Work out the finished part from the listing and answer in its coordinate system (mm). Face numbers are marked on the shaded views. A direction names the side the tool comes from. Coordinates: 2 decimals unless noted, no trailing zeros. Loops run counter-clockwise (first coordinate to the right, second up) from the corner with the lowest first, then second, coordinate; pieces in that order, holes last. Notation, with made-up numbers: (58, -39) -> (78, -39) arc R26 cw to (78, -13) -> close; hole circle Ø11 at (74, 45). An arc over 180 degrees is marked (long way). Answer as CSV lines item,"result".
Autodesk Fusion 360 part; units mm, degrees
sketch "Sketch1" plane through (0, 0, 0) normal (0, 0, 1) x (1, 0, 0)
  line L0 (49.35, -38.85) -> (-49.35, -38.85)
  line L1 (-49.35, -38.85) -> (-49.35, 38.85)
  line L2 (-49.35, 38.85) -> (49.35, 38.85)
  line L3 (49.35, 38.85) -> (49.35, -38.85)
  line L4 (49.35, -38.85) -> (-49.35, 38.85) construction
  line L5 (-49.35, -38.85) -> (49.35, 38.85) construction
  dimension "d1" = 98.7
  dimension "d2" = 77.7
extrude "Extrude1" add sketch "Sketch1" along normal blind 4
sketch "Sketch2" plane through (0, 0, 4) normal (0, 0, 1) x (-1, 0, 0)
  line L0 (-49.35, -38.85) -> (49.35, -38.85)
  line L1 (49.35, -38.85) -> (49.35, 38.85)
  line L2 (49.35, 38.85) -> (-49.35, 38.85)
  line L3 (-49.35, 38.85) -> (-49.35, -38.85)
  line L4 (35.35, -38.85) -> (-34.25, -38.85)
  line L5 (-34.25, -38.85) -> (-34.25, 9.95)
  line L6 (-34.25, 9.95) -> (35.35, 9.95)
  line L7 (35.35, 9.95) -> (35.35, -38.85)
  dimension "d5" = 69.6
  dimension "d6" = 48.8
  dimension "d7" = 14
extrude "Extrude2" add sketch "Sketch2" along normal blind 10 contours L0 L4 L5 L6 L7
sketch "Sketch3" plane through (0, 0, 14) normal (0, 0, 1) x (-1, 0, 0)
  line L0 (35.35, 9.95) -> (-34.25, 9.95)
  line L1 (-34.25, 9.95) -> (-34.25, -38.85)
  line L2 (-34.25, -38.85) -> (35.35, -38.85)
  line L3 (35.35, -38.85) -> (35.35, 9.95)
  line L4 (30.35, -38.85) -> (-28.35, -38.85)
  line L5 (-28.35, -38.85) -> (-28.35, 0.45)
  line L6 (-28.35, 0.45) -> (30.35, 0.45)
  line L7 (30.35, 0.45) -> (30.35, -38.85)
  dimension "d10" = 39.3
  dimension "d11" = 58.7
  dimension "d12" = 5
extrude "Extrude3" add sketch "Sketch3" along normal blind 20 contours L2 L4 L5 L6 L7
sketch "Sketch4" plane through (0, 0, 4) normal (0, 0, 1) x (-1, 0, 0)
  line L0 (-34.25, -38.85) -> (-34.25, 9.95)
  line L1 (-34.25, 9.95) -> (35.35, 9.95)
  line L2 (35.35, 9.95) -> (35.35, -38.85)
  line L3 (35.35, -38.85) -> (49.35, -38.85)
  line L4 (49.35, -38.85) -> (49.35, 38.85)
  line L5 (49.35, 38.85) -> (-49.35, 38.85)
  line L6 (-49.35, 38.85) -> (-49.35, -38.85)
  line L7 (-49.35, -38.85) -> (-34.25, -38.85)
  line L8 (47.35, 38.85) -> (37.35, 38.85)
  line L9 (37.35, 38.85) -> (37.35, 24.85)
  line L10 (37.35, 24.85) -> (47.35, 24.85)
  line L11 (47.35, 24.85) -> (47.35, 38.85)
  line L12 (33.35, 38.85) -> (16.35, 38.85)
  line L13 (16.35, 38.85) -> (16.35, 21.85)
  line L14 (16.35, 21.85) -> (33.35, 21.85)
  line L15 (33.35, 21.85) -> (33.35, 38.85)
  line L16 (13.35, 38.85) -> (0.35, 38.85)
  line L17 (0.35, 38.85) -> (0.35, 22.85)
  line L18 (0.35, 22.85) -> (13.35, 22.85)
  line L19 (13.35, 22.85) -> (13.35, 38.85)
  line L20 (-2.65, 38.85) -> (-15.65, 38.85)
  line L21 (-15.65, 38.85) -> (-15.65, 22.85)
  line L22 (-15.65, 22.85) -> (-2.65, 22.85)
  line L23 (-2.65, 22.85) -> (-2.65, 38.85)
  line L24 (-18.15, 38.85) -> (-34.15, 38.85)
  line L25 (-34.15, 38.85) -> (-34.15, 18.85)
  line L26 (-34.15, 18.85) -> (-18.15, 18.85)
  line L27 (-18.15, 18.85) -> (-18.15, 38.85)
  line L28 (-37.15, 38.85) -> (-45.15, 38.85)
  line L29 (-45.15, 38.85) -> (-45.15, 32.85)
  line L30 (-45.15, 32.85) -> (-37.15, 32.85)
  line L31 (-37.15, 32.85) -> (-37.15, 38.85)
  dimension "d15" = 10
  dimension "d16" = 14
  dimension "d17" = 17
  dimension "d18" = 17
  dimension "d19" = 2
  dimension "d20" = 4
  dimension "d21" = 13
  dimension "d22" = 16
  dimension "d23" = 13
  dimension "d24" = 16
  dimension "d25" = 3
  dimension "d26" = 3
  dimension "d27" = 16
  dimension "d28" = 20
  dimension "d29" = 2.5
  dimension "d30" = 8
  dimension "d31" = 6
  dimension "d32" = 3
extrude "Extrude4" add sketch "Sketch4" along normal blind 11 contours L5 L8 L9 L10 L11
extrude "Extrude5" add sketch "Sketch4" along normal blind 19 contours L5 L12 L13 L14 L15
extrude "Extrude6" add sketch "Sketch4" along normal blind 16 contours L5 L20 L21 L22 L23 | L5 L16 L17 L18 L19
extrude "Extrude7" add sketch "Sketch4" along normal blind 13.5 contours L5 L24 L25 L26 L27
extrude "Extrude8" add sketch "Sketch4" along normal blind 2 contours L5 L28 L29 L30 L31
sketch "Sketch5" plane through (0, -38.85, 0) normal (0, -1, 0) x (1, 0, 0)
  line L0 (-49.35, 0) -> (49.35, 0)
  line L1 (49.35, 0) -> (49.35, 4)
  line L2 (49.35, 4) -> (45.15, 4)
  line L3 (45.15, 4) -> (45.15, 6)
  line L4 (45.15, 6) -> (37.15, 6)
  line L5 (37.15, 6) -> (37.15, 4)
  line L6 (37.15, 4) -> (34.15, 4)
  line L7 (34.15, 4) -> (34.15, 17.5)
  line L8 (34.15, 17.5) -> (18.15, 17.5)
  line L9 (18.15, 17.5) -> (18.15, 4)
  line L10 (18.15, 4) -> (15.65, 4)
  line L11 (15.65, 4) -> (15.65, 20)
  line L12 (15.65, 20) -> (2.65, 20)
  line L13 (2.65, 20) -> (2.65, 4)
  line L14 (2.65, 4) -> (-0.35, 4)
  line L15 (-0.35, 4) -> (-0.35, 20)
  line L16 (-0.35, 20) -> (-13.35, 20)
  line L17 (-13.35, 20) -> (-13.35, 4)
  line L18 (-13.35, 4) -> (-16.35, 4)
  line L19 (-16.35, 4) -> (-16.35, 23)
  line L20 (-16.35, 23) -> (-33.35, 23)
  line L21 (-33.35, 23) -> (-33.35, 4)
  line L22 (-33.35, 4) -> (-37.35, 4)
  line L23 (-37.35, 4) -> (-37.35, 15)
  line L24 (-37.35, 15) -> (-47.35, 15)
  line L25 (-47.35, 15) -> (-47.35, 4)
  line L26 (-47.35, 4) -> (-49.35, 4)
  line L27 (-49.35, 4) -> (-49.35, 0)
  line L28 (-47.35, 4) -> (-37.35, 4)
  line L29 (-37.35, 4) -> (-37.35, 15)
  line L30 (-37.35, 15) -> (-47.35, 15)
  line L31 (-47.35, 15) -> (-47.35, 4)
  line L32 (-33.35, 4) -> (-16.35, 4)
  line L33 (-16.35, 4) -> (-16.35, 23)
  line L34 (-16.35, 23) -> (-33.35, 23)
  line L35 (-33.35, 23) -> (-33.35, 4)
  line L36 (-13.35, 4) -> (-0.35, 4)
  line L37 (-0.35, 4) -> (-0.35, 20)
  line L38 (-0.35, 20) -> (-13.35, 20)
  line L39 (-13.35, 20) -> (-13.35, 4)
  line L40 (2.65, 4) -> (15.65, 4)
  line L41 (15.65, 4) -> (15.65, 20)
  line L42 (15.65, 20) -> (2.65, 20)
  line L43 (2.65, 20) -> (2.65, 4)
  line L44 (18.15, 4) -> (34.15, 4)
  line L45 (34.15, 4) -> (34.15, 17.5)
  line L46 (34.15, 17.5) -> (18.15, 17.5)
  line L47 (18.15, 17.5) -> (18.15, 4)
  line L48 (37.15, 4) -> (45.15, 4)
  line L49 (45.15, 4) -> (45.15, 6)
  line L50 (45.15, 6) -> (37.15, 6)
  line L51 (37.15, 6) -> (37.15, 4)
extrude "Extrude9" add sketch "Sketch5" along normal blind 1 contours L23 L24 L25 L28 L29 L30 L31 | L3 L4 L5 L48 L49 L50 L51 | L19 L20 L21 L32 L33 L34 L35 | L7 L8 L9 L44 L45 L46 L47 | L15 L16 L17 L36 L37 L38 L39 | L11 L12 L13 L40 L41 L42 L43
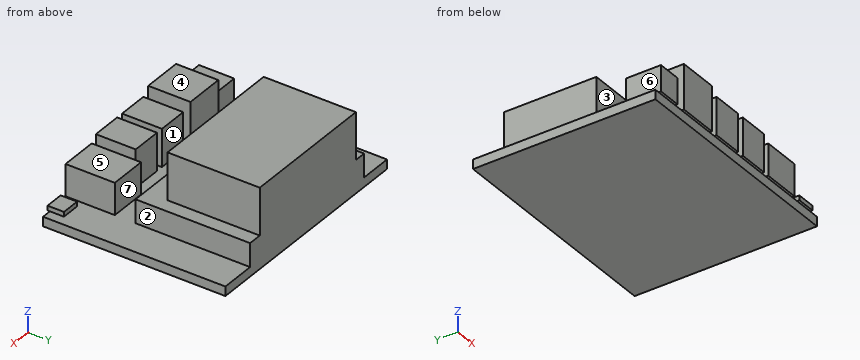
(1) A cutting plane is placed at D-D, the plane x = 38.5. Write down the section's boundary in (y, z).
Computed values:
outline,"(-39.85, 4) -> (-38.85, 4) -> (-38.85, 0) -> (38.85, 0) -> (38.85, 4) -> (-32.85, 4) -> (-32.85, 6) -> (-39.85, 6) -> close"
(2) Which of the six approach directions +Z, -Z, +X, -X, +Y, -Y give full straight-line access (tool end or side, diameter ignored) to the marked faces 4, 5, 6 and 7?
Computed values:
face 4,"+Z, +X, -X, -Y"
face 5,"+Z, +X, -Y"
face 6,"+Z, -X, +Y, -Y"
face 7,"+Z, +X, -X"
(3) A cutting plane is placed at B-B, the plane x = 23.5. Write down the section's boundary in (y, z), and give its area (3 significant figures).
Computed values:
outline,"(-39.85, 4) -> (-38.85, 4) -> (-38.85, 0) -> (38.85, 0) -> (38.85, 34) -> (-0.45, 34) -> (-0.45, 14) -> (-9.95, 14) -> (-9.95, 4) -> (-18.85, 4) -> (-18.85, 17.5) -> (-39.85, 17.5) -> close"
area,"1,870 mm2"
(4) Consider line 1 along X through (y, z) = (-22, 6); line 2 along Y through (x, z) = (20, 6); line 3 along Z through (x, y) = (-37, -28). Determine where each line is inside the solid, lowest interval first.
Computed values:
line 1,"-33.35 to -16.35, 18.15 to 34.15"
line 2,"-39.85 to -18.85, -9.95 to 38.85"
line 3,"0 to 4"
(5) Flat-ended cylindrical pins translate along their axes: pin 1 Ø5 at (y, z) = (-29.5, 11.5) entering from -X; pin 2 Ø1 at (y, z) = (-35, 5) entering from +X; pin 3 Ø1.5 at (y, z) = (23.5, 8.5) entering from -X. Find the tip coordinate at first contact, or state that the pin passes through.
Computed values:
pin 1,"x = -47.35"
pin 2,"x = 45.15"
pin 3,"x = -35.35"
(6) A cutting plane is placed at C-C, the plane y = 3.5. Write down the section's boundary in (x, z), and give its area (3 significant figures).
Computed values:
outline,"(-49.35, 0) -> (49.35, 0) -> (49.35, 4) -> (34.25, 4) -> (34.25, 14) -> (28.35, 14) -> (28.35, 34) -> (-30.35, 34) -> (-30.35, 14) -> (-35.35, 14) -> (-35.35, 4) -> (-49.35, 4) -> close"
area,"2,260 mm2"
(7) For a pull along X with two mould halves and no side action, classify the marked faces 1, 2 and 3 as pulls with the +X half, pulls with the -X half, needs draft (parallel to the pull), parting line crosses it, or undercut.
Computed values:
face 1,"undercut"
face 2,"pulls with the +X half"
face 3,"needs draft"
(8) A cutting plane is placed at A-A, the plane z = 11. Write down the section's boundary in (x, y), and give its area (3 significant figures).
Computed values:
outline,"(-47.35, -39.85) -> (-37.35, -39.85) -> (-37.35, -24.85) -> (-47.35, -24.85) -> close; (-35.35, -9.95) -> (34.25, -9.95) -> (34.25, 38.85) -> (-35.35, 38.85) -> close; (-33.35, -39.85) -> (-16.35, -39.85) -> (-16.35, -21.85) -> (-33.35, -21.85) -> close; (-13.35, -39.85) -> (-0.35, -39.85) -> (-0.35, -22.85) -> (-13.35, -22.85) -> close; (2.65, -39.85) -> (15.65, -39.85) -> (15.65, -22.85) -> (2.65, -22.85) -> close; (18.15, -39.85) -> (34.15, -39.85) -> (34.15, -18.85) -> (18.15, -18.85) -> close"
area,"4,630 mm2"
